Build history of the part. All positions in model axes, mm. A direction names the side the tool comes from. Coordinates: 2 decimals unless noted, no trailing zeros. Loops run counter-clockwise (first coordinate to the right, second up) from the corner with the lowest first, then second, coordinate; pieces in that order, holes last. Notation, with made-up numbers: (82.5, 67.5) - (133.5, 67.5) arc R20 cw to (133.5, 91.5) - close; hole circle Ø1 at (59, -1). An arc over 180 degrees is marked (long way). One line per item, written item: value.
```python
from build123d import *

# Parameters (mm, degrees)
F0_R     = 1.486134
F1_DEPTH = 1.5
F2_DEPTH = 2
F0_R_2   = 1.175
F3_DEPTH = 3
F0_W     = 0.498902
F0_H     = 3.899722
F0_W_2   = 0.498903
F4_DEPTH = 1.5
F5_R     = 1


with BuildPart() as f1:
    # F0 (on Top) → F1 (new body, symmetric)
    with BuildSketch(Plane.XY):
        with BuildLine():
            Line((9.956507, 9.285055), (10.191603, 7.715109))
            ThreePointArc((10.191603, 7.715109), (10.478158, 8.338993), (10.576356, 9.018481))
            ThreePointArc((10.576356, 9.018481), (7.15933, 11.192339), (6.638307, 7.17609))
            Line((6.638307, 7.17609), (6.424053, 8.606856))
            ThreePointArc((6.424053, 8.606856), (7.83697, 10.786197), (9.956507, 9.285055))
        make_face()
        with BuildLine():
            ThreePointArc((6.638307, 7.17609), (8.536307, 6.645627), (10.191603, 7.715109))
            Line((10.191603, 7.715109), (9.956507, 9.285055))
            ThreePointArc((9.956507, 9.285055), (7.83697, 10.786197), (6.424053, 8.606856))
            Line((6.424053, 8.606856), (6.638307, 7.17609))
        make_face()
        with Locations((8.176356, 9.018481)):
            Circle(F0_R, mode=Mode.SUBTRACT)
    extrude(amount=F1_DEPTH, both=True)

    # F0 (on Top) → F2 (join, symmetric)
    with BuildSketch(Plane.XY):
        with BuildLine():
            Line((-8.083594, 2.783208), (-7.783598, 2.783208))
            ThreePointArc((-7.783598, 2.783208), (-7.668552, 3.092999), (-7.379205, 3.252638))
            Line((-7.379205, 3.252638), (10.459818, 5.923991))
            Line((10.459818, 5.923991), (10.191603, 7.715109))
            ThreePointArc((10.191603, 7.715109), (8.536307, 6.645627), (6.638307, 7.17609))
            Line((6.638307, 7.17609), (6.861082, 5.688423))
            Line((6.861082, 5.688423), (-7.423694, 3.549311))
            ThreePointArc((-7.423694, 3.549311), (-7.895881, 3.288779), (-8.083594, 2.783208))
        make_face()
        with BuildLine():
            ThreePointArc((6.638307, 7.17609), (8.536307, 6.645627), (10.191603, 7.715109))
            Line((10.191603, 7.715109), (9.956507, 9.285055))
            ThreePointArc((9.956507, 9.285055), (7.83697, 10.786197), (6.424053, 8.606856))
            Line((6.424053, 8.606856), (6.638307, 7.17609))
        make_face()
        with Locations((8.176356, 9.018481)):
            Circle(F0_R, mode=Mode.SUBTRACT)
        with Locations((8.176356, 9.018481)):
            Circle(F0_R)
    extrude(amount=F2_DEPTH, both=True)

    # F0 (on Top) → F3 (join, symmetric)
    with BuildSketch(Plane.XY):
        with BuildLine():
            Line((8.067619, 1.983345), (-0.828579, 1.983345))
            Line((-0.828579, 1.983345), (-1.832268, 2.783208))
            Line((-1.832268, 2.783208), (-2.733431, 2.783208))
            Line((-2.733431, 2.783208), (-4.733298, 2.783208))
            Line((-4.733298, 2.783208), (-7.783598, 2.783208))
            Line((-7.783598, 2.783208), (-8.083594, 2.783208))
            Line((-8.083594, 2.783208), (-9.383528, 2.783208))
            ThreePointArc((-9.383528, 2.783208), (-10.232056, 2.431737), (-10.583528, 1.583208))
            Line((-10.583528, 1.583208), (-10.583528, -6.717112))
            ThreePointArc((-10.583528, -6.717112), (-10.349214, -7.282798), (-9.783528, -7.517112))
            Line((-9.783528, -7.517112), (-8.983085, -7.517112))
            Line((-8.983085, -7.517112), (-8.484182, -7.517112))
            Line((-8.484182, -7.517112), (-0.182472, -7.517112))
            Line((-0.182472, -7.517112), (0.316431, -7.517112))
            Line((0.316431, -7.517112), (7.116681, -7.517112))
            Line((7.116681, -7.517112), (7.615583, -7.517112))
            Line((7.615583, -7.517112), (8.467619, -7.517112))
            ThreePointArc((8.467619, -7.517112), (9.033304, -7.282798), (9.267619, -6.717112))
            Line((9.267619, -6.717112), (9.267619, 0.783345))
            ThreePointArc((9.267619, 0.783345), (8.916147, 1.631874), (8.067619, 1.983345))
        make_face()
        with Locations((-5.415644, -4.574013)):
            Circle(F0_R_2, mode=Mode.SUBTRACT)
        with Locations((4.104344, -4.574013)):
            Circle(F0_R_2, mode=Mode.SUBTRACT)
    extrude(amount=F3_DEPTH, both=True)

    # F0 (on Top) → F4 (join, symmetric)
    with BuildSketch(Plane.XY):
        with Locations((7.366132, -9.466973)):
            Rectangle(F0_W, F0_H)
        with Locations((0.066979, -9.466973)):
            Rectangle(F0_W_2, F0_H)
        with Locations((-8.733633, -9.466973)):
            Rectangle(F0_W_2, F0_H)
        with BuildLine():
            Line((-4.733298, 2.783208), (-2.733431, 2.783208))
            Line((-2.733431, 2.783208), (-2.733431, 3.142395))
            ThreePointArc((-2.733431, 3.142395), (-3.733365, 3.784402), (-4.733298, 3.142395))
            Line((-4.733298, 3.142395), (-4.733298, 2.783208))
        make_face()
    extrude(amount=F4_DEPTH, both=True)

    # F5
    f5_edges = [f1.edges().sort_by_distance(p)[0] for p in [
        (-8.733634, -11.416834, 1.5),
        (0.066979, -11.416834, 1.5),
        (7.366132, -11.416834, 1.5),
        (7.366132, -11.416834, -1.5),
        (0.066979, -11.416834, -1.5),
        (-8.733634, -11.416834, -1.5),
    ]]
    fillet(f5_edges, radius=F5_R)


solid = f1.part
```
Item 1: Cut at B-B, the plane x = -5.25. Write the cut outline in (y, z), then the cut area to 3 significant figures.
Check result:
outline: (-7.52, -3) - (-5.74, -3) - (-5.74, 3) - (-7.52, 3) - close; (-3.41, -3) - (2.78, -3) - (2.78, 3) - (-3.41, 3) - close; (3.57, -2) - (3.87, -2) - (3.87, 2) - (3.57, 2) - close
area: 49.1 mm^2
Item 2: Cut at A-A, the plane y = -8.5. Write the cut outline in (x, z), then the cut area to 3 significant figures.
Check result:
outline: (-8.98, -1.5) - (-8.48, -1.5) - (-8.48, 1.5) - (-8.98, 1.5) - close; (-0.18, -1.5) - (0.32, -1.5) - (0.32, 1.5) - (-0.18, 1.5) - close; (7.12, -1.5) - (7.62, -1.5) - (7.62, 1.5) - (7.12, 1.5) - close
area: 4.49 mm^2
Item 3: Cut at D-D, the plane y = -2.5. Write the cut outline in (x, z).
Check result:
outline: (-10.58, -3) - (9.27, -3) - (9.27, 3) - (-10.58, 3) - close
Item 4: Drop flat-ended pins along their axis: P1, Ø1, axis at x = -4, z = -2.5, coming from the -Y side; P2, Ø3, axis at x = -6, z = -1, coming from the +Y side; P3, Ø3.5, axis at y = -9, z = -0.5, coming from the +X side. Give the stop position or say it passes through.
Check result:
P1: stops at y = -7.52
P2: stops at y = 3.99
P3: stops at x = 9.06
Item 5: Tool access for faces 4 (the face through (9.268, -3, 0)), 5 (the face through (-4, 3, -1.5)), 6 (the face through (7.117, -9, 0)), 7 (the face through (7.22, 11.22, 0.02)), 8 (the face through (-1, -2, -3)): list every direction of +Z, -Z, +X, -X, +Y, -Y with a clear straight run to the whole face (end or side of a thin tool).
Check result:
face 4: +Z, -Z, +X, -Y
face 5: -Z, +X
face 6: +Z, -Z, -Y
face 7: +Z, -Z
face 8: -Z, +X, -X, +Y, -Y
Item 6: Probe probe 1 along Y at (x, z) = (4.75, -0.85); probe 2 along X at (y, z) = (0, -0.6); probe 3 along Y at (x, z) = (5, 1.85). List the from-to ranges inside material, lowest first. Write a range as from..to.
Check result:
probe 1: y = -7.52..-5.56, -3.59..1.98, 5.07..5.37
probe 2: x = -10.58..9.27
probe 3: y = -7.52..-5.33, -3.81..1.98, 5.11..5.41
Item 7: Cut at C-C, the plane z = -0.1. Give the number of separate pieces and of enclosed holes in the cut face, then the cut area to 3 significant figures.
Check result:
separate pieces: 1
enclosed holes: 2
area: 221 mm^2
Item 8: Pull direction Y, two halves, no side cores. Call faces 1 (the face through (-8.73, -11.12, 1.21)), 2 (the face through (-8.983, -9, 0)), 3 (the face through (3.172, -5.289, -0.042)): released by +Y, released by -Y, zero draft, split by the parting line, or undercut.
Check result:
face 1: released by -Y
face 2: zero draft
face 3: undercut
